from build123d import *

# Parameters (mm, degrees)
SKETCH_1_R          = 1.5
EXTRUDE_1_DEPTH     = 10
SKETCH_2_R          = 3.75
CUT_EXTRUDE_1_DEPTH = 10


with BuildPart() as part:
    # 草图1 → 凸台-拉伸1 (new body)
    with BuildSketch(Plane.XY):
        with BuildLine():
            Line((1.5, 19.943670675), (1.5, 22.5))
            Line((1.5, 22.5), (-1.5, 22.5))
            Line((-1.5, 22.5), (-1.5, 19.943670675))
            ThreePointArc((-1.5, 19.943670675), (-6.180339887, 19.021130326), (-10.509070008, 17.016446385))
            Line((-10.509070008, 17.016446385), (-12.011642685, 19.084560252))
            Line((-12.011642685, 19.084560252), (-14.438693668, 17.321204495))
            Line((-14.438693668, 17.321204495), (-12.936120991, 15.253090628))
            ThreePointArc((-12.936120991, 15.253090628), (-16.180339887, 11.755705046), (-18.504032463, 7.589517943))
            Line((-18.504032463, 7.589517943), (-20.935246125, 8.379467148))
            Line((-20.935246125, 8.379467148), (-21.862297108, 5.526297599))
            Line((-21.862297108, 5.526297599), (-19.431083446, 4.736348394))
            ThreePointArc((-19.431083446, 4.736348394), (-20, 0), (-19.431083446, -4.736348394))
            Line((-19.431083446, -4.736348394), (-21.862297108, -5.526297599))
            Line((-21.862297108, -5.526297599), (-20.935246125, -8.379467148))
            Line((-20.935246125, -8.379467148), (-18.504032463, -7.589517943))
            ThreePointArc((-18.504032463, -7.589517943), (-16.180339887, -11.755705046), (-12.936120991, -15.253090628))
            Line((-12.936120991, -15.253090628), (-14.438693668, -17.321204495))
            Line((-14.438693668, -17.321204495), (-12.011642685, -19.084560252))
            Line((-12.011642685, -19.084560252), (-10.509070008, -17.016446385))
            ThreePointArc((-10.509070008, -17.016446385), (-6.180339887, -19.021130326), (-1.5, -19.943670675))
            Line((-1.5, -19.943670675), (-1.5, -22.5))
            Line((-1.5, -22.5), (1.5, -22.5))
            Line((1.5, -22.5), (1.5, -19.943670675))
            ThreePointArc((1.5, -19.943670675), (6.180339887, -19.021130326), (10.509070008, -17.016446385))
            Line((10.509070008, -17.016446385), (12.011642685, -19.084560252))
            Line((12.011642685, -19.084560252), (14.438693668, -17.321204495))
            Line((14.438693668, -17.321204495), (12.936120991, -15.253090628))
            ThreePointArc((12.936120991, -15.253090628), (16.180339887, -11.755705046), (18.504032463, -7.589517943))
            Line((18.504032463, -7.589517943), (20.935246125, -8.379467148))
            Line((20.935246125, -8.379467148), (21.862297108, -5.526297599))
            Line((21.862297108, -5.526297599), (19.431083446, -4.736348394))
            ThreePointArc((19.431083446, -4.736348394), (20, 0), (19.431083446, 4.736348394))
            Line((19.431083446, 4.736348394), (21.862297108, 5.526297599))
            Line((21.862297108, 5.526297599), (20.935246125, 8.379467148))
            Line((20.935246125, 8.379467148), (18.504032463, 7.589517943))
            ThreePointArc((18.504032463, 7.589517943), (16.180339887, 11.755705046), (12.936120991, 15.253090628))
            Line((12.936120991, 15.253090628), (14.438693668, 17.321204495))
            Line((14.438693668, 17.321204495), (12.011642685, 19.084560252))
            Line((12.011642685, 19.084560252), (10.509070008, 17.016446385))
            ThreePointArc((10.509070008, 17.016446385), (6.180339887, 19.021130326), (1.5, 19.943670675))
        make_face()
        with Locations((0, 12.5)):
            Circle(SKETCH_1_R, mode=Mode.SUBTRACT)
        with Locations((10.825317547, -6.25)):
            Circle(SKETCH_1_R, mode=Mode.SUBTRACT)
        with Locations((-10.825317547, -6.25)):
            Circle(SKETCH_1_R, mode=Mode.SUBTRACT)
    extrude(amount=EXTRUDE_1_DEPTH)

    # 草图2 → 切除-拉伸1 (cut)
    with BuildSketch(Plane.XY):
        Circle(SKETCH_2_R)
    extrude(amount=CUT_EXTRUDE_1_DEPTH, mode=Mode.SUBTRACT)


solid = part.part
Source: CAD feature listing. Evaluate the final solid. Frame: model axes, mm. A direction names the side the tool comes from. Coordinates: 2 decimals unless noted, no trailing zeros. Order: outer loops, then holes, each group sorted by start corner. A loop starts at its lowest first (then second) coordinate and runs counter-clockwise, first axis right, second up. Notation, with made-up numbers: M 30.25,80 L 34.25,80 A22 ccw 34.25,114 Z; hole C 22.5,18 d6. An arc over 180 degrees is marked long. Write each question's results on one line, items separated by ' | '. Start each with the question number.
Item 1: Cut plane D-D (z = 4). Count the separate pieces of the cut face and the enclosed holes in it, and give its area (3 significant figures).
Item 2: Draft query along X for faces 1 (the face through (-20.63, -5.126, 4.93)), 2 (the face through (11.271, 18.065, 4.93)), 3 (the face through (13.677, 16.273, 4.93)). Return one class per face: pulls with the +X half, pulls with the -X half, needs draft (parallel to the pull), parting line crosses it, or undercut.
Item 3: Cut plane C-C (y = -6.25). Return loops of the section in (x, z).
Item 4: First-contact query: pin 1 Ø2 at (y, z) = (-21.5, 4.5) entering from +X; pin 2 Ø2 at (y, z) = (21.5, 6) entering from -X; pin 3 Ø4 at (y, z) = (-6, 7.5) entering from -X. Flat tips, straight axial feed; report the tip coordinate or a pass-through.
Item 5: Set-up query: faces 4 (the face through (-11.25, 18.036, 4.93)), 5 (the face through (1.5, -21, 5)), 6 (the face through (-19.74, -7.99, 4.93)), 7 (the face through (13.698, -16.302, 4.93)). Return all of +Z, -Z, +X, -X, +Y, -Y with unobstructed straight access to the full face (end or side cutting, diameter ignored); none if empty.
Item 6: Line query: probe 1 along Y at (x, z) = (0, 4.75); probe 2 along X at (y, z) = (-7.5, 6.25); probe 3 along Y at (x, z) = (-1, 4.75). Output: solid intervals per line, ascending.
Item 7: Cut plane A-A (y = 0). Return loops of the section in (x, z).
Item 8: Cut plane B-B (x = 0). Return loops of the section in (y, z), and give its area (3 significant figures).
Checked values:
1) separate pieces: 1 | enclosed holes: 4 | area: 1,270 mm2
2) face 1: pulls with the -X half | face 2: undercut | face 3: pulls with the +X half
3) outline: M -21.63,0 L -12.33,0 L -12.33,10 L -21.63,10 Z; M -9.33,0 L 9.33,0 L 9.33,10 L -9.33,10 Z; M 12.33,0 L 21.63,0 L 21.63,10 L 12.33,10 Z
4) pin 1: stops at x = 1.5 | pin 2: stops at x = -1.5 | pin 3: stops at x = -21.86
5) face 4: +Z, -Z, +Y | face 5: +Z, -Z, +X, -Y | face 6: +Z, -Z, -Y | face 7: +Z, -Z, +X
6) probe 1: y = -22.5 to -3.75, 3.75 to 11, 14 to 22.5 | probe 2: x = -21.22 to -11.65, -10 to 10, 11.65 to 21.22 | probe 3: y = -22.5 to -3.61, 3.61 to 11.38, 13.62 to 22.5
7) outline: M -20,0 L -3.75,0 L -3.75,10 L -20,10 Z; M 3.75,0 L 20,0 L 20,10 L 3.75,10 Z
8) outline: M -22.5,0 L -3.75,0 L -3.75,10 L -22.5,10 Z; M 3.75,0 L 11,0 L 11,10 L 3.75,10 Z; M 14,0 L 22.5,0 L 22.5,10 L 14,10 Z | area: 345 mm2
